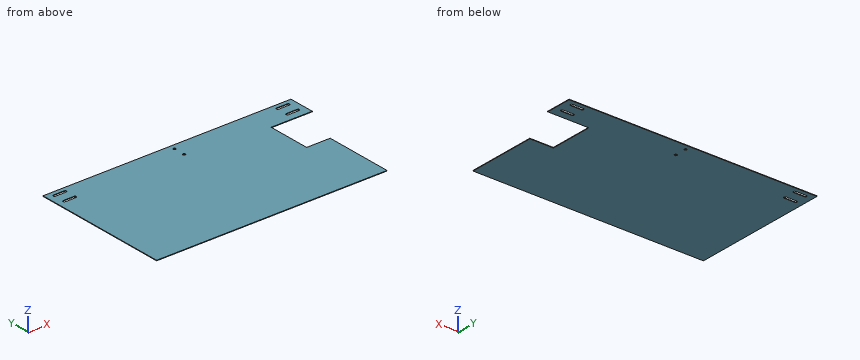
```python
from build123d import *

# Parameters (mm, degrees)
F0_R     = 6
F1_DEPTH = 2.5


with BuildPart() as f1:
    # F0 (on Top) → F1 (new body)
    with BuildSketch(Plane.XY):
        Polygon((0, 640), (0, 0), (1076, 0), (1076, 320), (966, 320), (966, 520), (1158, 520), (1158, 640), align=None)
        with BuildLine():
            ThreePointArc((33, 554), (27, 560), (33, 566))
            Line((33, 566), (83, 566))
            ThreePointArc((83, 566), (89, 560), (83, 554))
            Line((83, 554), (33, 554))
        make_face(mode=Mode.SUBTRACT)
        with BuildLine():
            ThreePointArc((33, 609), (27, 615), (33, 621))
            Line((33, 621), (83, 621))
            ThreePointArc((83, 621), (89, 615), (83, 609))
            Line((83, 609), (33, 609))
        make_face(mode=Mode.SUBTRACT)
        with Locations((593, 560)):
            Circle(F0_R, mode=Mode.SUBTRACT)
        with Locations((593, 615)):
            Circle(F0_R, mode=Mode.SUBTRACT)
        with BuildLine():
            ThreePointArc((1075, 554), (1069, 560), (1075, 566))
            Line((1075, 566), (1125, 566))
            ThreePointArc((1125, 566), (1131, 560), (1125, 554))
            Line((1125, 554), (1075, 554))
        make_face(mode=Mode.SUBTRACT)
        with BuildLine():
            ThreePointArc((1075, 609), (1069, 615), (1075, 621))
            Line((1075, 621), (1125, 621))
            ThreePointArc((1125, 621), (1131, 615), (1125, 609))
            Line((1125, 609), (1075, 609))
        make_face(mode=Mode.SUBTRACT)
    extrude(amount=F1_DEPTH)


solid = f1.part
```
Part model, mm, in its own coordinate system. Round coordinates to 2 decimals unless told otherwise and drop trailing zeros. Write each loop counter-clockwise with the first axis right and the second up, starting at its lowest first coordinate (ties: lowest second). Pieces come first, ordered by that corner, then holes. Notation, with made-up numbers: M 14.25,-6.75 L 67.25,-6.75 A22 ccw 67.25,29.25 Z; hole C 46.5,70 d7. An arc over 180 degrees is marked long. One line per question, with ' | ' between items.
(1) Probe line 1 along X through (y, z) = (615, 1.95); line 2 along Y through (x, z) = (593, 1.8); line 3 along Y through (x, z) = (1047.5, 1.65). List the from-to ranges inside material, lowest first.
Answer key:
line 1: x = 0 to 27, 89 to 587, 599 to 1069, 1131 to 1158 | line 2: y = 0 to 554, 566 to 609, 621 to 640 | line 3: y = 0 to 320, 520 to 640
(2) Pin check, flat tips, straight feed: pin 1 (6 mm diameter, centred on x = 787, y = 183, fed in from -Z); pin 2 (0.8 mm diameter, centred on x = 1097.5, z = 1.5, fed in from -Y). Stop position of each tip, or through.
Answer key:
pin 1: stops at z = 0 | pin 2: stops at y = 520
(3) Saw through at B-B on y = 194. Write the cut outline in (x, z).
Answer key:
outline: M 0,0 L 1076,0 L 1076,2.5 L 0,2.5 Z
(4) Saw through at C-C on y = 506. Write the cut outline in (x, z), then the cut area to 4 significant figures.
Answer key:
outline: M 0,0 L 966,0 L 966,2.5 L 0,2.5 Z | area: 2,415 mm^2
(5) Saw through at A-A on z = 1. Write the cut outline in (x, y).
Answer key:
outline: M 0,0 L 1076,0 L 1076,320 L 966,320 L 966,520 L 1158,520 L 1158,640 L 0,640 Z; hole M 33,554 L 83,554 A6 ccw 83,566 L 33,566 A6 ccw Z; hole M 33,609 L 83,609 A6 ccw 83,621 L 33,621 A6 ccw Z; hole C 593,560 d12; hole C 593,615 d12; hole M 1075,554 L 1125,554 A6 ccw 1125,566 L 1075,566 A6 ccw Z; hole M 1075,609 L 1125,609 A6 ccw 1125,621 L 1075,621 A6 ccw Z
